Autodesk Inventor part; units mm, degrees
ref_plane "Shim Holder Plane" through (0, 1, 0) normal (0, -1, 0) x (1, 0, 0)
ref_plane "YZ Plane" through (0, 0, 0) normal (1, 0, 0) x (0, 1, 0)
ref_plane "XZ Plane" through (0, 0, 0) normal (0, 1, 0) x (-1, 0, 0)
sketch "Main Platform" plane through (0, 0, 0) normal (0, 1, 0) x (-1, 0, 0)
  circle A0 centre (0, 0) radius 36
  dimension "d0" = 72
extrude "Main Platform Extrusion" add sketch "Main Platform" along normal blind 5
sketch "Main Hole" plane through (0, 0, 0) normal (0, -1, 0) x (1, 0, 0)
  circle A0 centre (0, 0) radius 36 construction
  circle A1 centre (0, 0) radius 10
  dimension "d3" = 20
extrude "Main Hole Cutout" cut sketch "Main Hole" against normal through all
sketch "Bottom Magnet Holes (MASTER)" plane through (0, 0, 0) normal (0, -1, 0) x (1, 0, 0)
  circle A0 centre (0, 0) radius 10 construction
  circle A1 centre (0, 0) radius 36 construction
  circle A2 centre (0, 0) radius 36 construction
  line L0 (0, -50.4) -> (0, 50.4) construction
  line L1 (0, 36) -> (0, -36) construction
  circle A3 centre (0, 0) radius 31 construction
  line L2 (0, 0) -> (26.8468, 15.5) construction
  line L3 (0, 0) -> (-26.8468, 15.5) construction
  line L4 (0, 0) -> (0, -31) construction
  dimension "d37" = 5
  dimension "d38" = 120
  dimension "d39" = 120
chamfer "Saline Well" distance 3.5 angle 30 1 edges at (-10, 5, 0) measured on face at (-27.0099, 5, -2.7674)
sketch "Top Magnet Holes" plane through (0, 5, 0) normal (0, 1, 0) x (1, 0, 0)
  circle A0 centre (0, 0) radius 31 construction
  point P0 (26.8468, -15.5)
  point P1 (-26.8468, -15.5)
  point P2 (0, 31)
ref_plane "Shim Holder Plane" through (0, 1, 0) normal (0, -1, 0) x (1, 0, 0)
sketch "Shim Holder" plane through (0, 1, 0) normal (0, -1, 0) x (1, 0, 0)
  circle A0 centre (0, 0) radius 36 construction
  circle A1 centre (0, 0) radius 13.5 construction
  circle A2 centre (0, 0) radius 15
  dimension "d137" = 30
extrude "Shim Holder Extrusion" add sketch "Shim Holder" against normal blind 1
sketch "Sketch22" plane through (0, 5, 0) normal (0, 1, 0) x (1, 0, 0)
  circle A0 centre (0, 0) radius 36 construction
  circle A1 centre (0, 0) radius 13.5 construction
  circle A2 centre (0, 0) radius 14.5
  circle A3 centre (0, 0) radius 36
  dimension "d110" = 1
extrude "Saline Well Recess" cut sketch "Sketch22" against normal blind 1.5
fillet "Fillet4" radius 1.5 1 edges at (-14.5, 5, 0)
hole "Top Magnet Recess" at (26.8468, 5, 15.5) at (0, 5, -31) at (-26.8468, 5, 15.5) direction (0, -1, 0) diameter 6.5 depth 2
hole "Bottom Magnet Recess" at (26.8468, 0, 15.5) at (0, 0, -31) at (-26.8468, 0, 15.5) direction (0, 1, 0) diameter 6.5 depth 0.5
chamfer "Chamfer6" distance 0.5 angle 45 9 edges at (36, 0, 0) (0, 0, -27.75) (26.8468, 0, 18.75) (-26.8468, 0, 18.75) (36, 3.5, 0) (-26.8468, 3.5, 12.25) (26.8468, 3.5, 12.25) (0, 3.5, -34.25) (-10, 0, 0)
sketch "Sketch25" plane through (0, 1, 0) normal (0, -1, 0) x (1, 0, 0)
  line L0 (-3, 5) -> (3, 5)
  line L1 (5, 3) -> (5, -3)
  line L2 (3, -5) -> (-3, -5)
  line L3 (-5, -3) -> (-5, 3)
  line L4 (-5, 5) -> (5, -5) construction
  line L5 (5, 5) -> (-5, -5) construction
  arc A0 (3, -5) -> (5, -3) centre (3, -3) ccw
  arc A1 (-5, -3) -> (-3, -5) centre (-3, -3) ccw
  arc A2 (-3, 5) -> (-5, 3) centre (-3, 3) ccw
  arc A3 (5, 3) -> (3, 5) centre (3, 3) ccw
  point P0 (0, 0)
  point P1 (0, 0)
  dimension "d140" = 10
  dimension "d141" = 10
  dimension "d142" = 2
extrude "Extrusion14" cut sketch "Sketch25" against normal through all
chamfer "Chamfer9" distance 1 angle 45 8 edges at (5, 2, 0) (4.4142, 2, 4.4142) (0, 2, 5) (-4.4142, 2, 4.4142) (-5, 2, 0) (-4.4142, 2, -4.4142) (0, 2, -5) (4.4142, 2, -4.4142)
properties part number "flat_platform_v1_mm"
Design review of the part built by this model. Coordinates are the model's own, in mm. A direction names the side the tool comes from. Give positions to 0.01 mm unless a question says otherwise; leave off trailing zeros. Return JSON: item names as keys, results as strings. Group by question number.
Item 1: Tool access review of faces 4 (the flat face through (0, 3.5, 15)), 5 (the flat face through (4, 1, 5)): name each direction out of +Z, -Z, +X, -X, +Y, -Y from which nothing blocks a thin tool from reaching the whole face with its end or side.
Item 2: Mouldability with a two-part tool opening along X and no side actions: class faces 1 (the conical face through (-4.68, 1.4, -4.71)), 2 (the flat face through (-7.4, 0, 8.4)), 3 (the flat face through (0, 3, -31)) as released by +X, released by -X, zero draft, split by the parting line, or undercut.
Item 3: Insertion check: pin 1 Ø3 at (x, z) = (1.5, -30) entering from +Y; pin 2 Ø7 at (x, z) = (0.5, -31) entering from -Y; pin 3 Ø6 at (x, z) = (26.85, 15.5) entering from +Y; pin 4 Ø6 at (x, z) = (1.5, 4.5) entering from -Y. Each pin has a flat end and moves straight along its axis. Give the tip position at first contact, or say it passes through.
Item 4: For probe 1 along Z at (x, y) = (0, 0.7); probe 2 along Z at (x, y) = (0, 3.05); probe 3 along Y at (x, z) = (1, -30), list the stretches that pass through material, from the lowest coordinate up.
Output:
{
 "1": {"face 4": "+Y", "face 5": "-Y"},
 "2": {"face 1": "undercut", "face 2": "zero draft", "face 3": "undercut"},
 "3": {"pin 1": "stops at y = 3.05", "pin 2": "stops at y = 0", "pin 3": "stops at y = 3", "pin 4": "stops at y = 1"},
 "4": {"probe 1": "z = -36 to -10, 10 to 36", "probe 2": "z = -35.95 to -34.3, -27.7 to -10.12, 10.12 to 35.95", "probe 3": "y = 0.5 to 3"}
}
